The drawing under review shows one solid part. Ordinate dimensions are in mm from its lowest x, y, z. Round coordinates to 2 decimals unless told otherwise and drop trailing zeros. Order: outer loops, then holes, each group sorted by start corner. A loop starts at its lowest first (then second) coordinate and runs counter-clockwise, first axis right, second up. Notation, with made-up numbers: (42, 13.25) -> (95, 13.25) arc R5 cw to (95, 18.25) -> close; hole circle Ø10 at (-16, 16.25). An arc over 180 degrees is marked (long way). Use a Markdown table: item, result. Add a question column.
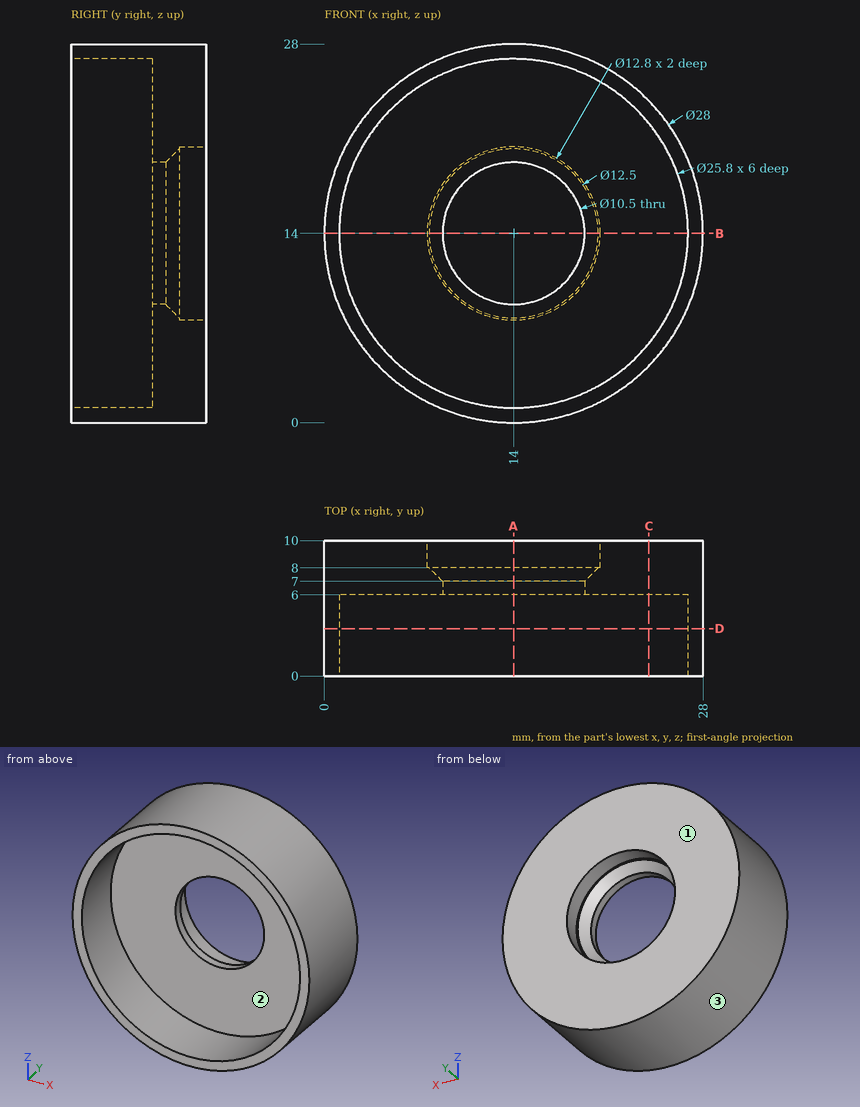
Q1. Draft analysis for pull direction Z (two halves, no side actions). For the marked faces 1, 2 and 3, state which applies: released by +Z, released by -Z, zero draft, split by the parting line, or undercut.
Q2. Add section C-C, the plane x = 24. Give the boundary of the cut face in (y, z), then the cut area to 3 significant figures.
Q3. To check wall thickness, follow line 1 along Z through (x, y) = (14, 3.8); line 2 along Z through (x, y) = (14, 9.35); line 3 along Y through (x, z) = (22.5, 12). State the ranges of each line that lie inside material, in increasing order.
Q4. Add section B-B, the plane z = 14. Give the boundary of the cut face in (x, y).
Q5. For pin 1 (6 mm diameter, centred on y = 7, z = 9, fed in from -X); pin 2 (4 mm diameter, centred on x = 17, z = 12, fed in from +Y); pin 3 (4 mm diameter, centred on x = 20.5, z = 10, fed in from -Y), all flat-tipped, find the tip position at first contact; note any pin that passes through.
Q6. Add section D-D, the plane y = 3.5. Give the boundary of the cut face in (x, z), then the cut area to 3 significant figures.
Q7. Add section A-A, the plane x = 14. Give the boundary of the cut face in (y, z), then the cut area to 3 significant figures.
Return value:
| question | item | result |
|---|---|---|
| 1 | face 1 | zero draft |
| 1 | face 2 | undercut |
| 1 | face 3 | split by the parting line |
| 2 | outline | (0, 4.2) -> (10, 4.2) -> (10, 23.8) -> (0, 23.8) -> (0, 22.15) -> (6, 22.15) -> (6, 5.85) -> (0, 5.85) -> close |
| 2 | area | 98.2 mm² |
| 3 | line 1 | 0 to 1.1, 26.9 to 28 |
| 3 | line 2 | 0 to 7.6, 20.4 to 28 |
| 3 | line 3 | 6 to 10 |
| 4 | outline | (0, 0) -> (1.1, 0) -> (1.1, 6) -> (8.75, 6) -> (8.75, 7) -> (7.75, 8) -> (7.6, 8) -> (7.6, 10) -> (0, 10) -> close; (19.25, 6) -> (26.9, 6) -> (26.9, 0) -> (28, 0) -> (28, 10) -> (20.4, 10) -> (20.4, 8) -> (20.25, 8) -> (19.25, 7) -> close |
| 5 | pin 1 | x = 0.14 |
| 5 | pin 2 | y = 7.36 |
| 5 | pin 3 | y = 6 |
| 6 | outline | circle Ø28 at (14, 14); hole circle Ø25.8 at (14, 14) |
| 6 | area | 93.0 mm² |
| 7 | outline | (0, 0) -> (10, 0) -> (10, 7.6) -> (8, 7.6) -> (8, 7.75) -> (7, 8.75) -> (6, 8.75) -> (6, 1.1) -> (0, 1.1) -> close; (0, 26.9) -> (6, 26.9) -> (6, 19.25) -> (7, 19.25) -> (8, 20.25) -> (8, 20.4) -> (10, 20.4) -> (10, 28) -> (0, 28) -> close |
| 7 | area | 77.6 mm² |
